from build123d import *

# Parameters (mm, degrees)
F1_DEPTH = 12
F2_R     = 2
F3_DEPTH = 25
F4_R     = 2
F5_DEPTH = 45
F6_R     = 5


with BuildPart() as f1:
    # F0 (on Right) → F1 (new body)
    with BuildSketch(Plane.YZ):
        Polygon((33, 0), (0, 0), (0, -16), (1.5, -16), (1.5, -1.5), (31.5, -1.5), (31.5, -16.072011), (33, -16), align=None)
    extrude(amount=F1_DEPTH)

    # F2 (on face) → F3 (cut)
    with BuildSketch(Plane.XY):
        with Locations((6, 16.5)):
            Circle(F2_R)
    extrude(amount=-F3_DEPTH, mode=Mode.SUBTRACT)

    # F4 (on face) → F5 (cut)
    with BuildSketch(Plane(origin=(0, 33, 0), x_dir=(-1, 0, 0), z_dir=(0, 1, 0))):
        with Locations((-6, -10)):
            Circle(F4_R)
    extrude(amount=-F5_DEPTH, mode=Mode.SUBTRACT)

    # F6
    f6_edges = [f1.edges().sort_by_distance(p)[0] for p in [
        (0, 32.25, -16.036005),
        (12, 32.25, -16.036005),
        (12, 0.75, -16),
        (0, 0.75, -16),
    ]]
    fillet(f6_edges, radius=F6_R)


solid = f1.part
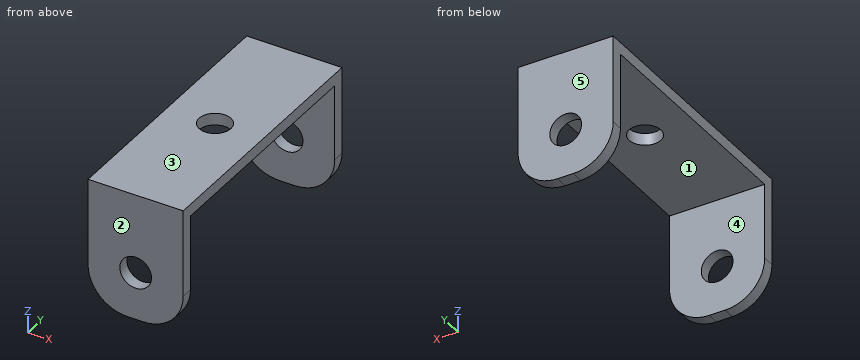
The listing builds one solid part. Answer for the finished solid, in the listing's coordinates (mm). Face numbers are marked on the shaded views. A direction names the side the tool comes from. Round coordinates to 2 decimals unless told otherwise and drop trailing zeros. Order: outer loops, then holes, each group sorted by start corner. A loop starts at its lowest first (then second) coordinate and runs counter-clockwise, first axis right, second up. Notation, with made-up numbers: (50.5, -7) -> (62.5, -7) arc R29 cw to (62.5, 30) -> close; hole circle Ø4 at (-7.75, 33.25). An arc over 180 degrees is marked (long way). Write each question's results on one line, items separated by ' | '. Start each with the question number.
Q1. Find section D-D (z = -6). Determine the outline of the cut face in (x, y).
Q2. Which of the six approach directions +Z, -Z, +X, -X, +Y, -Y give full straight-line access (tool end or side, diameter ignored) to the marked faces 4 and 5?
Q3. Find section A-A (z = -10). Determine the outline of the cut face in (x, y).
Q4. Each of these flat-tipped pins is pushed along its axis until it touches: pin 1 (1.6 mm diameter, centred on x = 6, y = 1, fed in from -Z); pin 2 (1 mm diameter, centred on x = 6.5, y = 16, fed in from -Z); pin 3 (6 mm diameter, centred on x = 5.5, y = 6, fed in from -Z). Where does it stop, or does it pass through?
Q5. Find section C-C (y = 16.5). Determine the outline of the cut face in (x, z), then the cut area to 3 significant figures.
Q6. The mould has two halves that part along Y. Classify the marked faces 1, 2 and 3: pulls with the +Y half, pulls with the -Y half, needs draft (parallel to the pull), parting line crosses it, or undercut.
Q7. Find section B-B (x = 6). Determine the outline of the cut face in (y, z).
Q8. Straight lines are drawn through the part: probe 1 along Y at (x, z) = (7, -6.25); probe 2 along Z at (x, y) = (6, 0.45); probe 3 along Z at (x, y) = (8.5, 17). For each, find the intervals that lie inside material, in ascending order. Write a range as from..to.
Worked answers:
1) outline: (0, 0) -> (12, 0) -> (12, 1.5) -> (0, 1.5) -> close; (0, 31.5) -> (12, 31.5) -> (12, 33) -> (0, 33) -> close
2) face 4: -Z, +X, -X | face 5: +Z, -Z, +X, -X, +Y
3) outline: (0, 0) -> (4, 0) -> (4, 1.5) -> (0, 1.5) -> close; (0, 31.5) -> (4, 31.5) -> (4, 33) -> (0, 33) -> close; (8, 0) -> (12, 0) -> (12, 1.5) -> (8, 1.5) -> close; (8, 31.5) -> (12, 31.5) -> (12, 33) -> (8, 33) -> close
4) pin 1: stops at z = -16 | pin 2: passes through | pin 3: stops at z = -1.5
5) outline: (0, -1.5) -> (4, -1.5) -> (4, 0) -> (0, 0) -> close; (8, -1.5) -> (12, -1.5) -> (12, 0) -> (8, 0) -> close | area: 12.0 mm2
6) face 1: undercut | face 2: pulls with the -Y half | face 3: needs draft
7) outline: (0, -16) -> (1.5, -16) -> (1.5, -12) -> (0, -12) -> close; (0, -8) -> (1.5, -8) -> (1.5, -1.5) -> (14.5, -1.5) -> (14.5, 0) -> (0, 0) -> close; (18.5, -1.5) -> (31.5, -1.5) -> (31.5, -8) -> (33, -8) -> (33, 0) -> (18.5, 0) -> close; (31.5, -16.07) -> (33, -16) -> (33, -12) -> (31.5, -12) -> close
8) probe 1: y = 0..1.5, 31.5..33 | probe 2: z = -16..-12, -8..0 | probe 3: z = -1.5..0
